The listing builds one solid part. Answer for the finished solid, in the listing's coordinates (mm). A direction names the side the tool comes from. Give positions to 0.01 mm unless a question says otherwise; leave off trailing zeros. Loops run counter-clockwise (first coordinate to the right, second up) from the corner with the lowest first, then second, coordinate; pieces in that order, holes last. Notation, with made-up numbers: (78, 52) - (106, 52) arc R19 cw to (106, 58) - close; hole circle Ø9 at (4.5, 83). An arc over 180 degrees is marked (long way). Answer in a Markdown table with one row per item. Add a question column.
```python
from build123d import *

# Parameters (mm, degrees)
SKETCH1_W               = 241.3
SKETCH1_H               = 254
BOSS_EXTRUDE1_DEPTH     = 6.35
SKETCH2_W               = 6.35
SKETCH2_H               = 12.7
CUT_EXTRUDE1_DEPTH      = 7.35
LPATTERN1_COUNT         = 10
LPATTERN1_PITCH         = 25.4
SKETCH3_W               = 12.7
SKETCH3_H               = 6.35
CUT_EXTRUDE2_DEPTH      = 7.35
LPATTERN2_COUNT         = 10
LPATTERN2_PITCH         = 25.4
SKETCH4_W               = 177.8
SKETCH4_H               = 190.5
CUT_EXTRUDE3_DEPTH      = 7.35
SKETCH5_W               = 101.6
SKETCH5_H               = 6.35
CUT_EXTRUDE4_DEPTH      = 7.35
CUT_EXTRUDE4_DEPTH_BACK = 76.2
FILLET1_R               = 6.35
SKETCH6_R               = 3.96875
CUT_EXTRUDE5_DEPTH      = 115.3


with BuildPart() as part:
    # Sketch1 → Boss-Extrude1 (new body)
    with BuildSketch(Plane(origin=(0, 0, 0), x_dir=(1, 0, 0), z_dir=(0, 1, 0))):
        with Locations((120.65, 127)):
            Rectangle(SKETCH1_W, SKETCH1_H)
    extrude(amount=BOSS_EXTRUDE1_DEPTH)

    # Sketch2 → Cut-Extrude1 (cut, through all)
    with BuildSketch(Plane(origin=(0, 6.35, 0), x_dir=(1, 0, 0), z_dir=(0, 1, 0))):
        with Locations((3.175, 6.35)):
            Rectangle(SKETCH2_W, SKETCH2_H)
        with Locations((238.125, 6.35)):
            Rectangle(SKETCH2_W, SKETCH2_H)
    cut_extrude1 = extrude(amount=-CUT_EXTRUDE1_DEPTH, mode=Mode.SUBTRACT)

    # LPattern1: Cut-Extrude1 ×10
    with Locations(*[(0, 0, -i * LPATTERN1_PITCH) for i in range(1, LPATTERN1_COUNT)]):
        add(cut_extrude1, mode=Mode.SUBTRACT)

    # Sketch3 → Cut-Extrude2 (cut, through all)
    with BuildSketch(Plane(origin=(0, 6.35, 0), x_dir=(1, 0, 0), z_dir=(0, 1, 0))):
        with Locations((6.35, 3.175)):
            Rectangle(SKETCH3_W, SKETCH3_H)
        with Locations((6.35, 250.825)):
            Rectangle(SKETCH3_W, SKETCH3_H)
    cut_extrude2 = extrude(amount=-CUT_EXTRUDE2_DEPTH, mode=Mode.SUBTRACT)

    # LPattern2: Cut-Extrude2 ×10
    with Locations(*[(i * LPATTERN2_PITCH, 0, 0) for i in range(1, LPATTERN2_COUNT)]):
        add(cut_extrude2, mode=Mode.SUBTRACT)

    # Sketch4 → Cut-Extrude3 (cut, through all)
    with BuildSketch(Plane(origin=(0, 6.35, 0), x_dir=(1, 0, 0), z_dir=(0, 1, 0))):
        with Locations((120.65, 127)):
            Rectangle(SKETCH4_W, SKETCH4_H)
    extrude(amount=-CUT_EXTRUDE3_DEPTH, mode=Mode.SUBTRACT)

    # Sketch5 → Cut-Extrude4 (cut, two sides)
    with BuildSketch(Plane(origin=(234.95, 0, 0), x_dir=(0, 0, -1), z_dir=(1, 0, 0))) as cut_extrude4_sk:
        with Locations((139.7, 3.175)):
            Rectangle(SKETCH5_W, SKETCH5_H)
    extrude(amount=CUT_EXTRUDE4_DEPTH, mode=Mode.SUBTRACT)
    extrude(cut_extrude4_sk.sketch, amount=-CUT_EXTRUDE4_DEPTH_BACK, mode=Mode.SUBTRACT)

    # Fillet1
    fillet1_edges = [part.edges().sort_by_distance(p)[0] for p in [
        (31.75, 3.175, -31.75),
        (31.75, 3.175, -222.25),
        (209.55, 3.175, -222.25),
        (209.55, 3.175, -31.75),
        (209.55, 3.175, -88.9),
        (209.55, 3.175, -190.5),
    ]]
    fillet(fillet1_edges, radius=FILLET1_R)

    # Sketch6 → Cut-Extrude5 (cut, through all)
    with BuildSketch(Plane.XZ.offset(107.95)):
        with Locations((174.625, -238.125)):
            Circle(SKETCH6_R)
    extrude(amount=-CUT_EXTRUDE5_DEPTH, mode=Mode.SUBTRACT)


solid = part.part
```
(1) A cutting plane is placed at C-C on z = -182. Determine the outline of the cut face in (x, y).
(2) A cutting plane is placed at A-A on z = -46.5. Determine the outline of the cut face in (x, y).
(3) A tool of negligible diameter and unlimited length cuts with its end or side. For faces 1 (the face through (127, 3, -3)), 2 (the face through (3, 3, -241.3)), 3 (the face through (234.95, 3, -9)), 4 (the face through (9, 3, -6.35)), from which of +Z, -Z, +X, -X, +Y, -Y can it reach the whole face along a straight path? Write none if from no direction.
(4) A cutting plane is placed at B-B on x = 58. Determine the outline of the cut face in (y, z).
(5) Given pin 1 Ø3 at (x, y) = (9, 4.5) entering from +Z; pin 2 Ø3 at (x, y) = (4, 2.5) entering from +Z; pin 3 Ø1.9 at (y, z) = (2, -4) entering from +X, each flat-ended and moving along its own axis, determine where each tip first touches the part or whether it passes through.
(6) The mould has two halves that part along Z. Classify faces 5 (the face through (3, 3, -152.4)), 6 (the face through (127, 3, -251)), 7 (the face through (238, 3, -25.4)), 8 (the face through (222, 3, 0)): pulls with the +Z half, pulls with the -Z half, needs draft (parallel to the pull), parting line crosses it, or undercut.
(7) Find the intervals of material crossed by line 1 along Z through (x, y) = (41, 5.5); line 2 along Z through (x, y) = (220.5, 2.5); line 3 along X through (y, z) = (4.75, -49), in increasing order. Write a range as [from, to].
Evaluation:
| question | item | result |
|---|---|---|
| 1 | outline | (6.35, 0) - (31.75, 0) - (31.75, 6.35) - (6.35, 6.35) - close |
| 2 | outline | (0, 0) - (31.75, 0) - (31.75, 6.35) - (0, 6.35) - close; (209.55, 0) - (241.3, 0) - (241.3, 6.35) - (209.55, 6.35) - close |
| 3 | face 1 | +Z, +Y, -Y |
| 3 | face 2 | -X, +Y, -Y |
| 3 | face 3 | +Z, +X, +Y, -Y |
| 3 | face 4 | +Z, -X, +Y, -Y |
| 4 | outline | (0, -247.65) - (6.35, -247.65) - (6.35, -222.25) - (0, -222.25) - close; (0, -31.75) - (6.35, -31.75) - (6.35, -6.35) - (0, -6.35) - close |
| 5 | pin 1 | stops at z = -6.35 |
| 5 | pin 2 | stops at z = -12.7 |
| 5 | pin 3 | stops at x = 228.6 |
| 6 | face 5 | undercut |
| 6 | face 6 | needs draft |
| 6 | face 7 | undercut |
| 6 | face 8 | pulls with the +Z half |
| 7 | line 1 | z = [-254, -222.25], [-31.75, 0] |
| 7 | line 2 | z = [-254, -190.5], [-88.9, 0] |
| 7 | line 3 | x = [0, 31.75], [209.55, 241.3] |
